The model under review builds one solid part; all positions refer to its coordinate system, in mm. Face numbers are marked on the shaded views. A direction names the side the tool comes from. Coordinates: 2 decimals unless noted, no trailing zeros. Loops run counter-clockwise (first coordinate to the right, second up) from the corner with the lowest first, then second, coordinate; pieces in that order, holes last. Notation, with made-up numbers: (-2, -8.5) - (42, -8.5) arc R11 cw to (42, 7.5) - close; hole circle Ø6 at (-6, -39). An arc over 180 degrees is marked (long way). One line per item, written item: value. Start each with the question number.
1. Insertion check: P1, Ø2, axis at y = -2, z = 4, coming from the +X side; P2, Ø3.5, axis at y = -6.5, z = 4, coming from the +X side; P3, Ø3.5, axis at y = -7.5, z = 4, coming from the -X side. Each pin has a flat end and moves straight along its axis. Give the tip position at first contact, or say it passes through.
2. We need section A-A, the plane x = -2. Give the boundary of the cut face in (y, z).
3. To check wall thickness, follow line 1 (X direction, y = -6.25, z = 4.55); line 2 (Y direction, x = 0.25, z = 0.35); line 3 (X direction, y = -3.25, z = 0.6). State the ranges of each line that lie inside material, in increasing order.
4. We need section C-C, the plane y = -5.5. Give the boundary of the cut face in (x, z).
5. We need section D-D, the plane x = 2.5. Give the boundary of the cut face in (y, z), then the cut area to 3 significant figures.
6. Mouldability with a two-part tool opening along Y and no side actions: class the marked faces 6, 7 and 8 as +Y half, -Y half, draft (parallel to the pull), parting line (faces both ways), or undercut.
7. For the marked faces 1, 2, 3, 4 and 5, list the 3-axis set-ups (+Z, -Z, +X, -X, +Y, -Y) from which the entire face can be reached by the end or side of a thin tool; tool diameter is ignored.
8. We need section B-B, the plane z = 1.85. Give the boundary of the cut face in (x, y), then the cut area to 3 significant figures.
from build123d import *

# Parameters (mm, degrees)
RESSALTO_EXTRUS_O1_DEPTH = 6


with BuildPart() as part:
    # Esboço1 → Ressalto-extrusão1 (new body)
    with BuildSketch(Plane.XY):
        with BuildLine():
            Line((-3, -5.228144515), (-3, -8.5))
            Line((-3, -8.5), (3, -8.5))
            Line((3, -8.5), (3, -5.228144515))
            Line((3, -5.228144515), (4.087420479, -4.721072019))
            ThreePointArc((4.087420479, -4.721072019), (3.647489335, -4.490964091), (3.194657217, -4.28741522))
            ThreePointArc((3.194657217, -4.28741522), (2.423308565, -4.011422259), (1.628622126, -3.812363669))
            ThreePointArc((1.628622126, -3.812363669), (0, -3.65195839), (-1.628622126, -3.812363669))
            ThreePointArc((-1.628622126, -3.812363669), (-2.423308565, -4.011422259), (-3.194657217, -4.28741522))
            ThreePointArc((-3.194657217, -4.28741522), (-3.647489335, -4.490964091), (-4.087420479, -4.721072019))
            Line((-4.087420479, -4.721072019), (-3, -5.228144515))
        make_face()
        with BuildLine():
            Line((-2.341083864, -0.230576635), (-1.628622126, -3.812363669))
            ThreePointArc((-1.628622126, -3.812363669), (0, -3.65195839), (1.628622126, -3.812363669))
            Line((1.628622126, -3.812363669), (2.341083864, -0.230576635))
            ThreePointArc((2.341083864, -0.230576635), (1.176205684, -0.05778328), (0, 0))
            ThreePointArc((0, 0), (-1.176205684, -0.05778328), (-2.341083864, -0.230576635))
        make_face()
    extrude(amount=RESSALTO_EXTRUS_O1_DEPTH)


solid = part.part
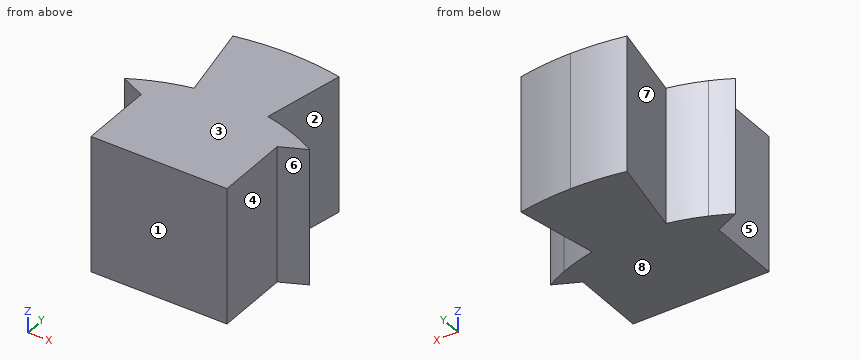
Findings below:
1. P1: x = 2.19
1. P2: x = 4.03
1. P3: x = -3
2. outline: (-8.5, 0) - (-3.9, 0) - (-3.9, 6) - (-8.5, 6) - close; (-1.95, 0) - (-0.17, 0) - (-0.17, 6) - (-1.95, 6) - close
3. line 1: -3 to 3
3. line 2: -8.5 to 0
3. line 3: -1.74 to 1.74
4. outline: (-3, 0) - (3, 0) - (3, 6) - (-3, 6) - close
5. outline: (-8.5, 0) - (-4.04, 0) - (-4.04, 6) - (-8.5, 6) - close
5. area: 26.8 mm2
6. face 6: -Y half
6. face 7: undercut
6. face 8: draft
7. face 1: +Z, -Z, +X, -X, -Y
7. face 2: +Z, -Z, +X
7. face 3: +Z, +X, -X, +Y, -Y
7. face 4: +Z, -Z, +X, -Y
7. face 5: +Z, -Z, -X, -Y
8. outline: (-4.09, -4.72) - (-3, -5.23) - (-3, -8.5) - (3, -8.5) - (3, -5.23) - (4.09, -4.72) arc R8.35 ccw to (1.63, -3.81) - (2.34, -0.23) arc R12 ccw to (-2.34, -0.23) - (-1.63, -3.81) arc R8.35 ccw to start
8. area: 43.7 mm2
